CAD build for the part. Positions are in the model's coordinates, mm. A direction names the side the tool comes from. Coordinates: 2 decimals unless noted, no trailing zeros. Loops run counter-clockwise (first coordinate to the right, second up) from the corner with the lowest first, then second, coordinate; pieces in that order, holes last. Notation, with made-up numbers: (-39, -15.5) -> (0, -15.5) arc R18 ccw to (0, 9.5) -> close; hole circle Ø8 at (7, -2). An arc over 180 degrees is marked (long way). Write each question's results on one line, items separated by ' | '.
Autodesk Inventor part; units mm, degrees
ref_plane "Work Plane1" through (1.525, 0, 0) normal (0, 0, 1) x (1, 0, 0)
ref_plane "YZ Plane" through (0, 0, 0) normal (1, 0, 0) x (0, 1, 0)
ref_plane "XZ Plane" through (0, 0, 0) normal (0, 1, 0) x (-1, 0, 0)
sketch "Boceto1" plane through (0, 0, 0) normal (0, 0, 1) x (1, 0, 0)
  line L0 (0, 2.95) -> (0, 2)
  line L1 (31, 2) -> (45, 2)
  line L2 (45, 2) -> (45, 0)
  line L3 (45, 0) -> (-0.4001, 0)
  line L4 (-9.4801, 0) -> (54.08, 0)
  line L5 (-0.4001, 0) -> (-0.4001, 2.95)
  line L6 (-0.4001, 2.95) -> (0, 2.95)
  line L7 (31, 2) -> (30.5705, 2)
  line L8 (30.5705, 2) -> (0, 2)
  line L9 (0, -0.59) -> (0, 3.54)
  dimension "d0" = 45
  dimension "d1" = 14
  dimension "d2" = 4
  dimension "d9" = 0.4001
  dimension "d10" = 5.9
  dimension "d13" = 0.4295
  dimension "d14" = 4
revolve "Cuerpo" add sketch "Boceto1" angle 360 about axis through (45, 0, 0) along (-1, 0, 0)
sketch "Boceto2" plane through (-0.4001, 0, 0) normal (-1, 0, 0) x (0, 0, 1)
  line L0 (0, 4.0415) -> (3.5, 2.0207)
  line L1 (3.5, 2.0207) -> (3.5, -2.0207)
  line L2 (3.5, -2.0207) -> (0, -4.0415)
  line L3 (0, -4.0415) -> (-3.5, -2.0207)
  line L4 (-3.5, -2.0207) -> (-3.5, 2.0207)
  line L5 (-3.5, 2.0207) -> (0, 4.0415)
  point P0 (0, 0)
  point P1 (0, 0)
  dimension "d11" = 7
extrude "Cabeza" add sketch "Boceto2" along normal blind 2.4
sketch "Boceto4" plane through (0, 0, 0) normal (0, 0, 1) x (1, 0, 0)
  line L0 (-2.8001, 3.5) -> (-2.8001, 4.0415)
  line L1 (-2.8001, 4.0415) -> (-2.4875, 4.0415)
  line L2 (-2.4875, 4.0415) -> (-2.8001, 3.5)
  line L3 (-3.2801, 0) -> (0.0799, 0)
  line L4 (-0.4001, 4.0415) -> (-2.8001, 4.0415)
  line L5 (-2.8001, 2.0207) -> (-2.8001, 4.0415)
  dimension "d5" = 30
  dimension "d19" = 7
revolve "Chaflán1" cut sketch "Boceto4" angle 360 about axis through (-10, 0, 0) along (1, 0, 0)
thread "Rosca"
chamfer "Chaflán2" distance 0.4294 distance2 0.4295 1 edges at (45, -2, 0) measured on face at (45, -0.2364, -0.6233)
ref_plane "Work Plane1" through (1.525, 0, 0) normal (0, 0, 1) x (1, 0, 0)
equation "\"d1\" = GEL"
equation "\"d2\" = GD"
equation "\"d10\" = SD2"
equation "\"d14\" = BDM"
equation "\"d11\" = SW"
equation "\"d3\" = KOH - SD"
equation "\"d5\" = ANG1"
equation "\"d19\" = SW0"
equation "\"d15\" = GEL"
equation "\"d6\" = -0.5 * SPD + 0.5 * GD"
equation "\"NLG\" = 25"
equation "\"GD\" = NND"
equation "\"BDM\" = NND"
equation "\"KOH\" = 2.8"
equation "\"GEL\" = 14"
equation "\"SW\" = 7"
equation "\"SW0\" = SW"
equation "\"SPD\" = NND - 1.2269 * PTC"
equation "\"SD2\" = SDH"
equation "\"SD\" = 0.4"
equation "\"ANG1\" = 30deg"
equation "\"GAL\" = 0.61345 * PTC"
equation "\"GUL\" = 0.61345 * PTC"
equation "\"RR\" = 0.15"
equation "\"WFT\" = RR"
equation "\"GD1\" = THREADDIA - 1.2269 * PTC"
equation "\"THREADDIA\" = 4"
equation "\"SDH\" = 5.9"
equation "\"TOA\" = 30deg"
equation "\"PTC\" = 0.7"
equation "\"NND\" = 4"
equation "\"E0\" = 1.155 * SW"
properties part number "UNI 5737 - M4 x 25" material "Acero, suave"
Q1. Cut at A-A on x = 39. Write the cut outline in (y, z), and give its area (3 significant figures).
Results are:
outline: circle Ø4 at (0, 0) | area: 12.6 mm^2
Q2. Drop flat-ended pins along their axis: pin 1 (4 mm diameter, centred on x = 39.5, z = -1, fed in from +Y); pin 2 (1.5 mm diameter, centred on x = 28.5, y = 1.5, fed in from -Z). Give the stop position or say it passes through.
Results are:
pin 1: y = 2 | pin 2: z = -1.85
Q3. Which spindle directions (+Z, -Z, +X, -X, +Y, -Y) get a long thin tool onto all of the face, cutting with end or side? Do faces 1 (the flat face through (-0.4, -3, -1)), 2 (the conical face through (-2.724, -3.632, 0.009)). Say none if no direction does.
Results are:
face 1: +X | face 2: -X, -Y
Q4. Wall check: L1, parallel to X at y = -2, z = 2.75; L2, parallel to X at y = -1, z = 2.5; L3, parallel to Y at x = 24, z = 1.25. Give the ranges that are in metal, low to high. Write a range as from..to.
Results are:
L1: -2.8..-0.4 | L2: -2.8..0 | L3: -1.56..1.56
